Here's how the part is built. I have some questions about the finished solid (model axes, mm). A direction names the side the tool comes from. Give positions to 0.01 mm unless a question says otherwise; leave off trailing zeros. Order: outer loops, then holes, each group sorted by start corner. A loop starts at its lowest first (then second) coordinate and runs counter-clockwise, first axis right, second up. Notation, with made-up numbers: M -23.5,-22.75 L 30.5,-22.75 A31 cw 30.5,16.25 Z; hole C 25,85.5 d9. An arc over 180 degrees is marked long. Use one line per item in the form item = value.
from build123d import *

# Parameters (mm, degrees)
SKETCH1_R           = 25
BOSS_EXTRUDE1_DEPTH = 29
CUT_EXTRUDE1_START  = -5
SKETCH2_R           = 25
SKETCH2_R_2         = 24
CUT_EXTRUDE1_DEPTH  = 5
SKETCH3_R           = 22
CUT_EXTRUDE2_DEPTH  = 27


with BuildPart() as part:
    # Sketch1 → Boss-Extrude1 (new body)
    with BuildSketch(Plane(origin=(0, 0, 0), x_dir=(1, 0, 0), z_dir=(0, 1, 0))):
        with Locations(Location((0, 0, 0), (0, 0, 270))):
            Circle(SKETCH1_R)
    extrude(amount=BOSS_EXTRUDE1_DEPTH)

    # Sketch2 → Cut-Extrude1 (cut)
    with BuildSketch(Plane(origin=(0, 29, 0), x_dir=(1, 0, 0), z_dir=(0, 1, 0)).offset(CUT_EXTRUDE1_START)):
        with Locations(Location((0, 0, 0), (0, 0, 270))):
            Circle(SKETCH2_R)
        with Locations(Location((0, 0, 0), (0, 0, 270))):
            Circle(SKETCH2_R_2, mode=Mode.SUBTRACT)
    extrude(amount=CUT_EXTRUDE1_DEPTH, mode=Mode.SUBTRACT)

    # Sketch3 → Cut-Extrude2 (cut)
    with BuildSketch(Plane(origin=(0, 29, 0), x_dir=(1, 0, 0), z_dir=(0, 1, 0))):
        with Locations(Location((0, 0, 0), (0, 0, 270))):
            Circle(SKETCH3_R)
    extrude(amount=-CUT_EXTRUDE2_DEPTH, mode=Mode.SUBTRACT)


solid = part.part
Q1. I want a section at A-A on x = 0. Write out the boundary of the cut face in (y, z), then the cut area to 3 significant figures.
Found:
outline = M 0,-25 L 24,-25 L 24,-24 L 29,-24 L 29,-22 L 2,-22 L 2,22 L 29,22 L 29,24 L 24,24 L 24,25 L 0,25 Z
area = 252 mm²
Q2. I need wall thicknesses on L1, parallel to X at y = 20.75, z = 0; L2, parallel to Y at x = 10, z = -15.5; L3, parallel to X at y = 11.5, z = -11. Which ranges of each line are inside material? Lowest first, please.
Found:
L1 = -25 to -22, 22 to 25
L2 = 0 to 2
L3 = -22.45 to -19.05, 19.05 to 22.45
Q3. I want a section at D-D on y = 25.25. Write out the boundary of the cut face in (x, z).
Found:
outline = C 0,0 d48; hole C 0,0 d44
Q4. On a 3-axis mill with a long thin cutter (end or side, diameter ignored), from which of +Z, -Z, +X, -X, +Y, -Y can I reach the whole of each face in a straight line? I mean faces 1 (the face through (7.21, 26.46, 22.89)), 2 (the face through (-21.2, 29, 7)). Say none if no direction works.
Found:
face_1 = +Y
face_2 = +Z, -Z, +X, -X, +Y
Q5. I want a section at B-B on z = 0. Write out the boundary of the cut face in (x, y).
Found:
outline = M -25,0 L 25,0 L 25,24 L 24,24 L 24,29 L 22,29 L 22,2 L -22,2 L -22,29 L -24,29 L -24,24 L -25,24 Z
Q6. I'm going to push flat-ended pins straight in: pin 1 Ø1 at (x, y) = (-3, 10.5) entering from -Z; pin 2 Ø2 at (x, y) = (-4.5, 5) entering from -Z; pin 3 Ø4 at (y, z) = (24, -16.5) entering from -X; pin 4 Ø5 at (x, z) = (-2, -2.5) entering from -Y. Where does each tip first touch, or does it pass through?
Found:
pin_1 = -24.87
pin_2 = -24.75
pin_3 = -20.37
pin_4 = 0
Q7. Thinking about a two-plate mould opening in X: for faces 3 (the face through (7.509, 11.832, 23.846)), 4 (the face through (0, 0, 0)), 5 (the face through (-21.477, 15.689, -4.769)), which applies, +X half, -X half, draft (parallel to the pull), parting line (faces both ways), or undercut?
Found:
face_3 = parting line
face_4 = draft
face_5 = undercut
Q8. I want a section at C-C on y = 13.75. Write out the boundary of the cut face in (x, z), then the cut area to 3 significant figures.
Found:
outline = C 0,0 d50; hole C 0,0 d44
area = 443 mm²
